Autodesk Inventor part; units mm, degrees
ref_plane "YZ Plane" through (0, 0, 0) normal (1, 0, 0) x (0, 1, 0)
ref_plane "XZ Plane" through (0, 0, 0) normal (0, 1, 0) x (-1, 0, 0)
ref_plane "XY Plane" through (0, 0, 0) normal (0, 0, 1) x (1, 0, 0)
sketch "스케치1" plane through (0, 0, 0) normal (0, 0, 1) x (1, 0, 0)
  circle A0 centre (2, 0) radius 7.45
  line L0 (0, 0) -> (2, 0)
  circle A1 centre (0, 0) radius 4
  line L1 (-2.6458, -3) -> (2.6458, -3)
  dimension "d1" = 14.9
  dimension "d2" = 2
  dimension "d3" = 8
  dimension "d4" = 3
extrude "돌출1" add sketch "스케치1" along normal blind 5 contours A0 | A1 L1 | L1 A1
extrude "돌출2" add sketch "스케치1" against normal blind 3.5 contours A1 L1 picked at (1.0912, -0.393)
sketch "스케치3" plane through (2, 0, 0) normal (0, 0, -1) x (-1, 0, 0)
  arc A0 (4.6458, -3) -> (-0.6458, -3) centre (2, 0) ccw construction
  line L0 (-0.6458, -3) -> (4.6458, -3) construction
  circle A1 centre (2, 0) radius 5
  dimension "d12" = 10
extrude "돌출3" add sketch "스케치3" along normal blind 1
properties part number "감속기어1 - 상단 편심축"
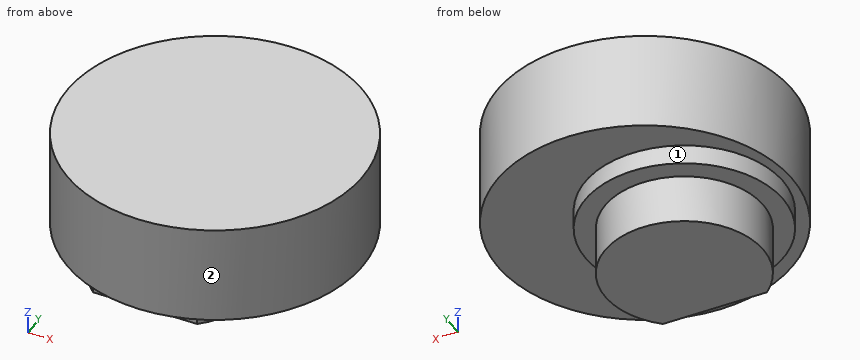
CAD build for the part. Positions are in the model's coordinates, mm. Face numbers are marked on the shaded views. A direction names the side the tool comes from. Round coordinates to 2 decimals unless told otherwise and drop trailing zeros. Order: outer loops, then holes, each group sorted by start corner. A loop starts at its lowest first (then second) coordinate and runs counter-clockwise, first axis right, second up.
Item 1: Tool access for the marked faces 1 and 2: list every direction of +Z, -Z, +X, -X, +Y, -Y with a clear straight run to the whole face (end or side of a thin tool).
Item 2: Pin check, flat tips, straight feed: pin 1 (1.5 mm diameter, centred on y = -4, z = 1, fed in from +X); pin 2 (1.2 mm diameter, centred on x = 0.5, z = -2, fed in from -Y); pin 3 (2 mm diameter, centred on x = 5.5, z = 3, fed in from -Y). Stop position of each tip, or through.
Item 3: Saw through at C-C on z = 0.75. Write the cut outline in (x, y).
Item 4: Saw through at D-D on x = 4.75. Write the cut outline in (y, z).
Item 5: Saw through at A-A on y = 0. Write the cut outline in (x, z).
Item 6: Saw through at B-B on x = -1.25. Write the cut outline in (y, z).
Item 7: Probe line 1 along X through (y, z) = (3, -2.5); line 2 along Z through (x, y) = (0.5, 6); line 3 along Y through (x, z) = (4.75, 3.75). List the from-to ranges inside material, lowest first.
Reported:
1. face 1: -Z
1. face 2: +Z, -Z
2. pin 1: stops at x = 8.7
2. pin 2: stops at y = -3
2. pin 3: stops at y = -7.02
3. outline: circle Ø14.9 at (2, 0)
4. outline: (-6.92, 0) - (-1.56, 0) - (-1.56, -1) - (1.56, -1) - (1.56, 0) - (6.92, 0) - (6.92, 5) - (-6.92, 5) - close
5. outline: (-5.45, 0) - (-5, 0) - (-5, -1) - (-4, -1) - (-4, -3.5) - (4, -3.5) - (4, -1) - (5, -1) - (5, 0) - (9.45, 0) - (9.45, 5) - (-5.45, 5) - close
6. outline: (-6.7, 0) - (-4.84, 0) - (-4.84, -1) - (-3, -1) - (-3, -3.5) - (3.8, -3.5) - (3.8, -1) - (4.84, -1) - (4.84, 0) - (6.7, 0) - (6.7, 5) - (-6.7, 5) - close
7. line 1: x = -2.65 to 2.65
7. line 2: z = 0 to 5
7. line 3: y = -6.92 to 6.92
